```python
from build123d import *

# Parameters (mm, degrees)
BOSS_EXTRUDE1_DEPTH = 2
SKETCH2_R           = 3.5
SKETCH2_R_2         = 2.5
BOSS_EXTRUDE2_DEPTH = 2


with BuildPart() as part:
    # Sketch1 → Boss-Extrude1 (new body)
    with BuildSketch(Plane.XY):
        with BuildLine():
            Line((-0.981334679, -13.192307692), (-3.434671375, -0.673076923))
            ThreePointArc((-3.434671375, -0.673076923), (0, 3.5), (3.434671375, -0.673076923))
            Line((3.434671375, -0.673076923), (0.981334679, -13.192307692))
            ThreePointArc((0.981334679, -13.192307692), (0, -14), (-0.981334679, -13.192307692))
        make_face()
    extrude(amount=BOSS_EXTRUDE1_DEPTH)

    # Sketch2 → Boss-Extrude2 (add)
    with BuildSketch(Plane.XY.offset(2)):
        Circle(SKETCH2_R)
        Circle(SKETCH2_R_2, mode=Mode.SUBTRACT)
    extrude(amount=BOSS_EXTRUDE2_DEPTH)


solid = part.part
```
Build history of the part. All positions in model axes, mm. Give positions to 0.01 mm unless a question says otherwise; leave off trailing zeros. Order: outer loops, then holes, each group sorted by start corner. A loop starts at its lowest first (then second) coordinate and runs counter-clockwise, first axis right, second up. Notation, with made-up numbers: M 18,-31.75 L 45,-31.75 A22 cw 45,2.25 Z; hole C -27.75,89.25 d1. An arc over 180 degrees is marked long. Return JSON: item names as keys, results as strings.
Q1. Wall check: probe 1 along Y at (x, z) = (0, 2.75); probe 2 along Z at (x, y) = (0.5, 2); probe 3 along X at (y, z) = (1, 2.7). Give the ranges that are in metal, low to high. Write a range as from..to.
Answer list:
{"probe 1": "y = -3.5..-2.5, 2.5..3.5", "probe 2": "z = 0..2", "probe 3": "x = -3.35..-2.29, 2.29..3.35"}
Q2. Two-plate mould, pull along X, no slides. Class faces 1 (the face through (0, 0, 2)), 2 (the face through (-2.19, -7.02, 0.99)), 3 (the face through (-0.54, -2.44, 2.99)), 4 (the face through (2.225, -6.845, 0.986)): pulls with the +X half, pulls with the -X half, needs draft (parallel to the pull), parting line crosses it, or undercut.
Answer list:
{"face 1": "undercut", "face 2": "pulls with the -X half", "face 3": "undercut", "face 4": "pulls with the +X half"}
Q3. Band-saw the part on B-B (x = 0). Give the cut face in (y, z), then the cut area to 3 significant figures.
Answer list:
{"outline": "M -14,0 L 3.5,0 L 3.5,4 L 2.5,4 L 2.5,2 L -2.5,2 L -2.5,4 L -3.5,4 L -3.5,2 L -14,2 Z", "area": "39.0 mm^2"}
Q4. Band-saw the part on D-D (z = 0.5). Give the cut face in (x, y), then the cut area to 3 significant figures.
Answer list:
{"outline": "M -3.43,-0.67 L -0.98,-13.19 A1 ccw 0.98,-13.19 L 3.43,-0.67 A3.5 ccw long Z", "area": "80.4 mm^2"}
Q5. Band-saw the part on A-A (z = 2.2). Give the cut face in (x, y), then the cut area to 3 significant figures.
Answer list:
{"outline": "C 0,0 d7; hole C 0,0 d5", "area": "18.8 mm^2"}
Q6. Flat gauge pins, fed straight in: pin 1 (1 mm diameter, centred on y = -3.5, z = 1.5, fed in from +X); pin 2 (1.5 mm diameter, centred on x = 1, y = 1, fed in from +Z). Where does each tip first touch, or does it go through?
Answer list:
{"pin 1": "stops at x = 2.98", "pin 2": "stops at z = 2"}
Q7. Band-saw the part on C-C (y = 0). Give the cut face in (x, z).
Answer list:
{"outline": "M -3.5,0 L 3.5,0 L 3.5,4 L 2.5,4 L 2.5,2 L -2.5,2 L -2.5,4 L -3.5,4 Z"}
